Geometry: final body of the model. Coordinates: model frame, mm. A direction names the side the tool comes from. Give positions to 0.01 mm unless a question says otherwise; leave off trailing zeros. Loops run counter-clockwise (first coordinate to the right, second up) from the corner with the lowest first, then second, coordinate; pieces in that order, holes last. Notation, with made-up numbers: (30.25, 10.5) -> (71.25, 10.5) arc R13 cw to (71.25, 18.5) -> close; hole circle Ø1 at (7, -0.5). An arc over 180 degrees is marked (long way). Answer in a Markdown table with one row per item. Add a question column.
1) First-contact query: P1, Ø2, axis at x = -2.5, z = -1, coming from the +Y side; P2, Ø8, axis at y = 9, z = 54, coming from the +X side; P3, Ø4, axis at y = 6, z = 23.5, coming from the -X side; P4, Ø6, axis at x = 1, y = 6.5, coming from the +Z side. Flat tips, straight axial feed; report the tip coordinate or a pass-through.
2) Line query: line 1 (Z direction, x = 13, y = 3); line 2 (Z direction, x = 0, y = -6.5); line 3 (Y direction, x = 0, z = 66.5) (3 decimals). Output: solid intervals per line, ascending. Write a range as from..to.
3) Access query for faces 1 (the cylindrical face through (-14.125, 5.856, 59.901)), 2 (the cylindrical face through (15.77, 4.97, 27.34)), 3 (the cylindrical face through (-0.708, 3.186, -18.335)), 4 (the flat face through (9.5, -3, 66.548)), 5 (the flat face through (-7.48, -7.43, 60.16)). Directions: +Z, -Z, +X, -X, +Y, -Y. A direction counts if a zero-diameter tool reaches every point of the face in a straight line with its end or side. Return the directions, or none.
4) Draft query along X for faces 6 (the flat face through (-10.2, -3.3, -5.969)), 7 (the conical face through (5.414, -1.705, 63.901)), 8 (the cylindrical face through (-7.056, -13.566, 0.773)). Return one class per face: +X half, -X half, draft (parallel to the pull), parting line (faces both ways), or undercut.
5) Section query A-A (z = 27). Return the cut outline in (x, y), plus the area to 3 significant figures.
```python
from build123d import *

# Parameters (mm, degrees)
SKETCH1_R          = 16.5354
EXTRUDE1_DEPTH     = 66.548
CHAMFER1_SIZE      = 0.762
SKETCH6_R          = 15.6845
EXTRUDE2_DEPTH     = 5.969
SKETCH7_W          = 20.828
SKETCH7_H          = 10.31875
CUT_EXTRUDE4_DEPTH = 19.84248
HOLE1_D            = 5.0038
HOLE1_DEPTH        = 4.7498
CIRPATTERN1_COUNT  = 4


with BuildPart() as part:
    # Sketch1 → Extrude1 (new body)
    with BuildSketch(Plane.XY):
        Circle(SKETCH1_R)
    extrude(amount=EXTRUDE1_DEPTH)

    # Sketch2 → Cut-Revolve1 (revolve, cut)
    with BuildSketch(Plane(origin=(0, 0, 0), x_dir=(1, 0, 0), z_dir=(0, 1, 0)), mode=Mode.PRIVATE) as cut_revolve1_sk:
        Polygon((16.5354, -66.548), (16.5354, -52.6034), (15.2908, -53.848), (15.2908, -66.548), align=None)
    revolve(cut_revolve1_sk.sketch.rotate(Axis((0, 0, 0), (0, 0, 1)), 180), axis=Axis((0, 0, 0), (0, 0, 1)), mode=Mode.SUBTRACT)  # turned: the seam where the file's is

    # Sketch3 → Cut-Revolve2 (revolve, cut)
    with BuildSketch(Plane(origin=(0, 0, 0), x_dir=(1, 0, 0), z_dir=(0, 1, 0)), mode=Mode.PRIVATE) as cut_revolve2_sk:
        Polygon((15.2908, 0), (15.2908, -1.524), (16.5354, -2.7686), (16.5354, 0), align=None)
    revolve(cut_revolve2_sk.sketch.rotate(Axis((0, 0, 0), (0, 0, -1)), 180), axis=Axis((0, 0, 0), (0, 0, -1)), mode=Mode.SUBTRACT)  # turned: the seam where the file's is

    # S2D0002 → Cut-Revolve3 (revolve, cut)
    with BuildSketch(Plane(origin=(0, 0, 0), x_dir=(1, 0, 0), z_dir=(0, 1, 0))):
        Polygon((6.1849, -66.294), (9.525, -66.294), (9.525, -66.548), (0, -66.548), (0, -52.324), (4.9784, -52.324), (4.9784, -63.077393135), (5.642306865, -63.7413), align=None)
    revolve(axis=Axis((0, 0, 14.6685), (0, 0, -1)), mode=Mode.SUBTRACT)

    # Chamfer1
    chamfer1_edges = [part.edges().sort_by_distance(p)[0] for p in [
        (15.2908, 0, 66.548),
    ]]
    chamfer(chamfer1_edges, length=CHAMFER1_SIZE)

    # Sketch6 → Extrude2 (add)
    with BuildSketch(Plane(origin=(0, 0, 0), x_dir=(-1, 0, 0), z_dir=(0, 0, -1))):
        Circle(SKETCH6_R)
    extrude(amount=EXTRUDE2_DEPTH)

    # Sketch7 → Revolve1 (revolve)
    with BuildSketch(Plane(origin=(0, 0, 0), x_dir=(0, 0, -1), z_dir=(1, 0, 0)), mode=Mode.PRIVATE) as revolve1_sk:
        with Locations((16.383, -5.159375)):
            Rectangle(SKETCH7_W, SKETCH7_H)
    revolve(revolve1_sk.sketch.rotate(Axis((0, 0, 0), (0, 0, -1)), 270), axis=Axis((0, 0, 0), (0, 0, -1)))  # turned: the seam where the file's is

    # S2D0001 → Cut-Revolve5 (revolve, cut)
    with BuildSketch(Plane(origin=(0, 0, 0), x_dir=(1, 0, 0), z_dir=(0, 1, 0))):
        Polygon((3.2639, 24.861260017), (3.2639, 11.9888), (0, 11.9888), (0, 26.797), (4.3815, 26.797), align=None)
    revolve(axis=Axis((0, 0, 31.308359971), (0, 0, -1)), mode=Mode.SUBTRACT)

    # Sketch9 → Cut-Revolve6 (revolve, cut)
    with BuildSketch(Plane(origin=(0, 0, 0), x_dir=(0, -1, 0), z_dir=(1, 0, 0)), mode=Mode.PRIVATE) as cut_revolve6_sk:
        with BuildLine():
            Line((-10.31875, 19.3802), (-10.033, 20.1422))
            Line((-10.033, 20.1422), (-10.033, 25.781))
            ThreePointArc((-10.033, 25.781), (-9.932678675, 26.324796865), (-9.644922533, 26.797))
            Line((-9.644922533, 26.797), (-10.31875, 26.797))
            Line((-10.31875, 26.797), (-10.31875, 19.3802))
        make_face()
    revolve(cut_revolve6_sk.sketch.rotate(Axis((0, 0, -12.65936), (0, 0, -1)), 90), axis=Axis((0, 0, -12.65936), (0, 0, -1)), mode=Mode.SUBTRACT)  # turned: the seam where the file's is

    # Sketch13 → Cut-Extrude4 (cut, symmetric)
    with BuildSketch(Plane(origin=(0, 0, 0), x_dir=(1, 0, 0), z_dir=(0, 1, 0))):
        Polygon((8.5852, 26.797), (8.5852, 21.844), (10.033, 20.3962), (10.033, 26.797), align=None)
        Polygon((-8.5852, 26.797), (-8.5852, 21.844), (-10.033, 20.3962), (-10.033, 26.797), align=None)
    extrude(amount=CUT_EXTRUDE4_DEPTH, both=True, mode=Mode.SUBTRACT)

    # Hole1
    with Locations(Plane(origin=(-10.81222837, 10.81222837, 60.198), x_dir=(0.707106781, 0.707106781, 0), z_dir=(-0.707106781, 0.707106781, 0))):
        with Locations((0, 0)):
            hole1 = Hole(HOLE1_D / 2, depth=HOLE1_DEPTH)

    # CirPattern1: Hole1 ×4 about axis
    cirpattern1_axis = Axis((0, 0, 0), (0, 0, 1))
    for i in range(1, CIRPATTERN1_COUNT):
        add(hole1.rotate(cirpattern1_axis, i * 360 / CIRPATTERN1_COUNT), mode=Mode.SUBTRACT)


solid = part.part
```
Evaluation:
| question | item | result |
|---|---|---|
| 1 | P1 | y = 15.61 |
| 1 | P2 | x = 15.68 |
| 1 | P3 | x = -16.04 |
| 1 | P4 | z = 66.55 |
| 2 | line 1 | -5.97..66.55 |
| 2 | line 2 | -26.8..66.29 |
| 2 | line 3 | -14.577..-9.525, 9.525..14.577 |
| 3 | face 1 | +Z |
| 3 | face 2 | +Z, -Z |
| 3 | face 3 | -Z |
| 3 | face 4 | +Z, +X, -X, +Y, -Y |
| 3 | face 5 | none |
| 4 | face 6 | draft |
| 4 | face 7 | undercut |
| 4 | face 8 | parting line |
| 5 | outline | circle Ø33.07 at (0, 0) |
| 5 | area | 859 mm² |
